Work out the finished part from the listing and answer in its coordinate system (mm). Round coordinates to 2 decimals unless told otherwise and drop trailing zeros. Order: outer loops, then holes, each group sorted by start corner. A loop starts at its lowest first (then second) coordinate and runs counter-clockwise, first axis right, second up. Notation, with made-up numbers: (57, -17) - (113, -17) arc R7 cw to (113, -13) - close; hole circle Ø10 at (61, 15). An arc over 180 degrees is marked (long way). Answer in a Markdown table with one row per item.
from build123d import *

# Parameters (mm, degrees)
CYLINDER012_R     = 4
CYLINDER012_DEPTH = 4
CYLINDER013_R     = 2
CYLINDER013_DEPTH = 11.5
CYLINDER010_R     = 4
CYLINDER010_DEPTH = 4
CYLINDER011_R     = 2
CYLINDER011_DEPTH = 11.5
BOX002_W          = 15
BOX002_H          = 55
BOX002_DEPTH      = 4.5


with BuildPart() as cylinder015:
    # Cylinder012 → Cylinder012 (new body)
    with BuildSketch(Plane.XY.offset(7.5)):
        Circle(CYLINDER012_R)
    extrude(amount=CYLINDER012_DEPTH)


with BuildPart() as bolt_hole4_distance:
    # Cylinder013 → Cylinder013 (new body)
    with BuildSketch(Plane.XY):
        Circle(CYLINDER013_R)
    extrude(amount=CYLINDER013_DEPTH)

    # Fusion006: union Cylinder015
    add(cylinder015.part)


with BuildPart() as bolt_hole4_distance_1:
    # Fusion006 placement: moved
    add(bolt_hole4_distance.part.moved(Location((28, 45, -9))))


with BuildPart() as cylinder014:
    # Cylinder010 → Cylinder010 (new body)
    with BuildSketch(Plane.XY.offset(7.5)):
        Circle(CYLINDER010_R)
    extrude(amount=CYLINDER010_DEPTH)


with BuildPart() as bolt_hole3_distance:
    # Cylinder011 → Cylinder011 (new body)
    with BuildSketch(Plane.XY):
        Circle(CYLINDER011_R)
    extrude(amount=CYLINDER011_DEPTH)

    # Fusion005: union Cylinder014
    add(cylinder014.part)


with BuildPart() as bolt_hole3_distance_1:
    # Fusion005 placement: moved
    add(bolt_hole3_distance.part.moved(Location((28, 12, -9))))


with BuildPart() as z_distance:
    # Box002 → Box002 (new body)
    with BuildSketch(Plane(origin=(20.5, 0, -9), x_dir=(1, 0, 0), z_dir=(0, 0, 1))):
        with Locations((7.5, 27.5)):
            Rectangle(BOX002_W, BOX002_H)
    extrude(amount=BOX002_DEPTH)

    # Cut012: cut bolt-hole3-distance
    add(bolt_hole3_distance_1.part, mode=Mode.SUBTRACT)

    # Cut013: cut bolt-hole4-distance
    add(bolt_hole4_distance_1.part, mode=Mode.SUBTRACT)


with BuildPart() as z_distance_1:
    # Cut013 placement: moved
    add(z_distance.part.moved(Location((0, 0, -0.5))))


solid = z_distance_1.part
1) Find section C-C, the plane z = -8.95. Give the vertices of the cut face in (x, y).
Filled in:
| item | result |
|---|---|
| outline | (20.5, 0) - (35.5, 0) - (35.5, 55) - (20.5, 55) - close; hole circle Ø4 at (28, 12); hole circle Ø4 at (28, 45) |
2) Find the intervals of material crossed by probe 1 along Y at (x, z) = (28, -6.5); probe 2 along X at (y, z) = (12, -6.6); probe 3 along Y at (x, z) = (26.25, -8), in increasing order. Write a range as from..to.
Filled in:
| item | result |
|---|---|
| probe 1 | y = 0..10, 14..43, 47..55 |
| probe 2 | x = 20.5..26, 30..35.5 |
| probe 3 | y = 0..11.03, 12.97..44.03, 45.97..55 |
3) Find section B-B, the plane y = 45. Give the vertices of the cut face in (x, z), then the cut area to 3 significant figures.
Filled in:
| item | result |
|---|---|
| outline | (20.5, -9.5) - (26, -9.5) - (26, -5) - (20.5, -5) - close; (30, -9.5) - (35.5, -9.5) - (35.5, -5) - (30, -5) - close |
| area | 49.5 mm^2 |
4) Find section A-A, the plane x = 28. Give the vertices of the cut face in (y, z).
Filled in:
| item | result |
|---|---|
| outline | (0, -9.5) - (10, -9.5) - (10, -5) - (0, -5) - close; (14, -9.5) - (43, -9.5) - (43, -5) - (14, -5) - close; (47, -9.5) - (55, -9.5) - (55, -5) - (47, -5) - close |
5) The mould has two halves that part along Y. Classify faces 1 (the face through (29.908, 12.601, -7.281)), 2 (the face through (28, 28, -5)), 3 (the face through (28, 0, -7)): released by +Y, released by -Y, zero draft, split by the parting line, or undercut.
Filled in:
| item | result |
|---|---|
| face 1 | undercut |
| face 2 | zero draft |
| face 3 | released by -Y |
